```python
from build123d import *

# Parameters (mm, degrees)
F1_DEPTH = 7.62
F2_W     = 12.7
F2_H     = 5.9424509318
F3_ANGLE = 20
F5_DEPTH = 25.4
F7_DEPTH = 25.4


with BuildPart() as f1:
    # F0 (on Front) → F1 (new body)
    with BuildSketch(Plane.XZ):
        Polygon((15.875, -3.6650325341), (0, 0), (0, -19.622516), (15.875, -15.9574834659), align=None)
        Polygon((31.75, 0), (15.875, -3.6650325341), (15.875, -15.9574834659), (31.75, -19.622516), align=None)
    extrude(amount=F1_DEPTH)

    # F2 (on face) → F3 (revolve, cut)
    with BuildSketch(Plane.XZ.offset(7.62)):
        with Locations((9.525, -9.811258)):
            Rectangle(F2_W, F2_H)
        Polygon((15.875, -12.7824834659), (3.175, -12.7824834659), (3.175, -15.7145094932), align=None)
        Polygon((3.175, -3.9080065068), (3.175, -6.8400325341), (15.875, -6.8400325341), align=None)
    revolve(axis=Axis((15.875, -7.62, -9.811258), (0, 0, -1)), revolution_arc=F3_ANGLE, mode=Mode.SUBTRACT)

    # F4 (on face) → F5 (cut)
    with BuildSketch(Plane(origin=(0, 0, 0), x_dir=(-1, 0, 0), z_dir=(0, 1, 0))):
        Polygon((0, -19.622516), (0, 0), (-15.875, -3.6650325341), (-31.75, 0), (-31.75, -19.622516), (-15.875, -15.9574834659), align=None)
        Polygon((-15.875, -15.1754397357), (-30.988, -18.6645507082), (-30.988, -0.9579652918), (-15.875, -4.4470762643), (-0.762, -0.9579652918), (-0.762, -18.6645507082), align=None, mode=Mode.SUBTRACT)
    extrude(amount=-F5_DEPTH, mode=Mode.SUBTRACT)

    # F6 (on face) → F7 (cut)
    with BuildSketch(Plane.XZ.offset(7.62)):
        with BuildLine():
            Line((0.762, -9.811258), (0.762, -12.8777229028))
            ThreePointArc((0.762, -12.8777229028), (1.7932958238, -11.4961033935), (2.159, -9.811258))
            Line((2.159, -9.811258), (0.762, -9.811258))
        make_face()
        with BuildLine():
            Line((0.762, -6.7447930972), (0.762, -9.811258))
            Line((0.762, -9.811258), (2.159, -9.811258))
            ThreePointArc((2.159, -9.811258), (1.7932958238, -8.1264126065), (0.762, -6.7447930972))
        make_face()
    extrude(amount=-F7_DEPTH, mode=Mode.SUBTRACT)


solid = f1.part
```
Source: CAD feature listing. Evaluate the final solid. Frame: model axes, mm. A direction names the side the tool comes from. Give positions to 0.01 mm unless a question says otherwise; leave off trailing zeros. Write each loop counter-clockwise with the first axis right and the second up, starting at its lowest first coordinate (ties: lowest second). Pieces come first, ordered by that corner, then holes.
1. Access query for faces 1 (the face through (23.537, -3.757, -2.678)), 2 (the face through (16, 0, -10)), 3 (the face through (9.531, -6.517, -5.353)), 4 (the face through (8.213, -3.757, -16.944)). Directions: +Z, -Z, +X, -X, +Y, -Y. A direction counts if a zero-diameter tool reaches every point of the face in a straight line with its end or side. Return the directions, or none.
2. Section query B-B (y = -1.75). Return the cut outline in (x, z) (3 decimals), then the cut area to 3 significant figures.
3. Section query D-D (x = 16.5). Return the cut outline in (y, z), then the cut area to 3 significant figures.
4. Section query C-C (z = -11). Return the cut outline in (x, y) (3 decimals).
5. Material intervals for line 1 along Z through (x, y) = (6, -3.75); line 2 along Z through (x, y) = (19.5, -5.5); line 3 along Y through (x, z) = (4.5, -9.25), sorted ascending.
6. Pull-direction query (Y, two-part tool) for faces 5 (the face through (19, -7.62, -10)), 6 (the face through (8.424, -3.757, -2.727)), 7 (the face through (9.706, -6.548, -14.228)); classes: +Y half, -Y half, draft (parallel to the pull), parting line (faces both ways), or undercut.
7. Section query A-A (z = -16.25). Return the cut outline in (x, y).
Output values:
1. face 1: +Z, +Y, -Y
1. face 2: +Z, -Z, +X, -X, +Y
1. face 3: none
1. face 4: -Z, +Y, -Y
2. outline: (0.762, -18.665) - (15.875, -15.175) - (30.988, -18.665) - (30.988, -0.958) - (15.875, -4.447) - (0.762, -0.958) - (0.762, -6.745) arc R4.064 cw to (0.762, -12.878) - close
2. area: 424 mm2
3. outline: (-7.62, -15.32) - (0, -15.32) - (0, -4.3) - (-7.62, -4.3) - close
3. area: 83.9 mm2
4. outline: (1.981, -7.62) - (3.175, -7.62) arc R12.7 cw to (3.941, -3.276) - (15.875, -7.62) - (30.988, -7.62) - (30.988, 0) - (1.981, 0) - close
5. line 1: z = -17.46 to -2.17
5. line 2: z = -16.01 to -3.61
5. line 3: y = -3.48 to 0
6. face 5: -Y half
6. face 6: draft
6. face 7: undercut
7. outline: (0.76, -7.62) - (11.22, -7.62) - (11.22, 0) - (0.76, 0) - close; (20.53, -7.62) - (30.99, -7.62) - (30.99, 0) - (20.53, 0) - close
